CAD build for the part. Positions are in the model's coordinates, mm. A direction names the side the tool comes from. Coordinates: 2 decimals unless noted, no trailing zeros. Loops run counter-clockwise (first coordinate to the right, second up) from the corner with the lowest first, then second, coordinate; pieces in that order, holes last. Notation, with made-up numbers: (82.25, 78.25) -> (117.25, 78.25) arc R17 ccw to (117.25, 104.25) -> close; hole circle Ø4 at (75.25, 18.25). An arc over 180 degrees is marked (long way). Write each question's results on one line, items separated by ' | '.
```python
from build123d import *

# Parameters (mm, degrees)
CROQUIS1_R              = 21
SALIENTE_EXTRUIR1_DEPTH = 1.5
CROQUIS2_R              = 18.9
SALIENTE_EXTRUIR2_DEPTH = 10.8
CROQUIS3_R              = 21
SALIENTE_EXTRUIR3_DEPTH = 1.5
CROQUIS8_R              = 12.5
SALIENTE_EXTRUIR5_DEPTH = 6.5
CROQUIS6_R              = 2
CORTAR_EXTRUIR3_DEPTH   = 36.973462441
CROQUIS5_R              = 2
CORTAR_EXTRUIR2_DEPTH   = 36.973462498
CROQUIS4_R              = 4
CORTAR_EXTRUIR1_DEPTH   = 36.973462441


with BuildPart() as part:
    # Croquis1 → Saliente-Extruir1 (new body)
    with BuildSketch(Plane.XY):
        Circle(CROQUIS1_R)
    extrude(amount=SALIENTE_EXTRUIR1_DEPTH)

    # Croquis2 → Saliente-Extruir2 (add)
    with BuildSketch(Plane.XY.offset(1.5)):
        with Locations(Location((0, 0, 0), (0, 0, 180))):
            Circle(CROQUIS2_R)
    extrude(amount=SALIENTE_EXTRUIR2_DEPTH)

    # Croquis3 → Saliente-Extruir3 (add)
    with BuildSketch(Plane.XY.offset(12.3)):
        Circle(CROQUIS3_R)
    extrude(amount=SALIENTE_EXTRUIR3_DEPTH)

    # Croquis8 → Saliente-Extruir5 (add)
    with BuildSketch(Plane.XY.offset(13.8)):
        with Locations(Location((0, 0, 0), (0, 0, 180))):
            Circle(CROQUIS8_R)
    extrude(amount=SALIENTE_EXTRUIR5_DEPTH)

    # Croquis6 → Cortar-Extruir3 (cut, through all)
    with BuildSketch(Plane(origin=(0, 0, 0), x_dir=(1, 0, 0), z_dir=(0, 1, 0))):
        with Locations(Location((0, -17.5, 0), (0, 0, 270))):
            Circle(CROQUIS6_R)
    extrude(amount=-CORTAR_EXTRUIR3_DEPTH, mode=Mode.SUBTRACT)

    # Croquis5 → Cortar-Extruir2 (cut, through all)
    with BuildSketch(Plane(origin=(0, 0, 0), x_dir=(0, 0, -1), z_dir=(1, 0, 0))):
        with Locations(Location((-17.5, 0, 0), (0, 0, 180))):
            Circle(CROQUIS5_R)
    extrude(amount=-CORTAR_EXTRUIR2_DEPTH, mode=Mode.SUBTRACT)

    # Croquis4 → Cortar-Extruir1 (cut, through all)
    with BuildSketch(Plane.XY.offset(20.3)):
        Circle(CROQUIS4_R)
    extrude(amount=-CORTAR_EXTRUIR1_DEPTH, mode=Mode.SUBTRACT)


solid = part.part
```
Q1. Pull direction Z, two halves, no side cores. Call faces 1 (the flat face through (3, -3, 20.3)), 2 (the cylindrical face through (0.088, -7.921, 15.502)), 3 (the flat face through (4.4, 0.3, 0)): +Z half, -Z half, draft (parallel to the pull), parting line (faces both ways), or undercut.
Results are:
face 1: +Z half | face 2: undercut | face 3: -Z half
Q2. Drop flat-ended pins along their axis: pin 1 (12.5 mm diameter, centred on x = 0, y = 7, fed in from -Z); pin 2 (3.5 mm diameter, centred on x = 0, z = 17.5, fed in from +Y); pin 3 (1 mm diameter, centred on y = -3, z = 13, fed in from -X); pin 4 (3 mm diameter, centred on x = -4.5, z = 17.5, fed in from +Y). Give the stop position or say it passes through.
Results are:
pin 1: z = 0 | pin 2: y = 12.5 | pin 3: x = -20.85 | pin 4: y = 12.13
Q3. Which spindle directions (+Z, -Z, +X, -X, +Y, -Y) get a long thin tool onto all of the face, cutting with end or side? Do faces 4 (the flat face through (9, -9, 13.8)), 5 (the cylindrical face through (-7.919, -0.088, 15.502)), 6 (the cylindrical face through (-18.027, -5.677, 6.824)). Say none if no direction does.
Results are:
face 4: +Z | face 5: -X | face 6: none
Q4. Cut at C-C on z = 17.5. Write the cut outline in (x, y).
Results are:
outline: (-12.34, -2) arc R12.5 ccw to (-2, -12.34) -> (-2, -3.46) arc R4 cw to (-3.46, -2) -> close; (-12.34, 2) -> (-3.46, 2) arc R4 cw (long way) to (2, -3.46) -> (2, -12.34) arc R12.5 ccw (long way) to start
Q5. Cut at D-D on x = -5.5. Write the cut outline in (y, z).
Results are:
outline: (-20.27, 0) -> (20.27, 0) -> (20.27, 1.5) -> (18.08, 1.5) -> (18.08, 12.3) -> (20.27, 12.3) -> (20.27, 13.8) -> (11.22, 13.8) -> (11.22, 20.3) -> (-11.22, 20.3) -> (-11.22, 13.8) -> (-20.27, 13.8) -> (-20.27, 12.3) -> (-18.08, 12.3) -> (-18.08, 1.5) -> (-20.27, 1.5) -> close; hole circle Ø4 at (0, 17.5)
Q6. Wall check: L1, parallel to Y at x = 0, z = 5; L2, parallel to Z at x = -15.5, y = 12; L3, parallel to Z at x = 0, y = -7.5. Give the ranges that are in metal, low to high. Write a range as from..to.
Results are:
L1: -18.9..-4, 4..18.9 | L2: 0..1.5, 12.3..13.8 | L3: 0..15.5, 19.5..20.3
Q7. Cut at A-A on y = 0. Write the cut outline in (x, z), and give its area (3 significant figures).
Results are:
outline: (-21, 0) -> (-4, 0) -> (-4, 15.5) -> (-12.5, 15.5) -> (-12.5, 13.8) -> (-21, 13.8) -> (-21, 12.3) -> (-18.9, 12.3) -> (-18.9, 1.5) -> (-21, 1.5) -> close; (-12.5, 19.5) -> (-4, 19.5) -> (-4, 20.3) -> (-12.5, 20.3) -> close; (4, 0) -> (21, 0) -> (21, 1.5) -> (18.9, 1.5) -> (18.9, 12.3) -> (21, 12.3) -> (21, 13.8) -> (12.5, 13.8) -> (12.5, 20.3) -> (4, 20.3) -> close | area: 500 mm^2
